For this review, take the finished solid that the model builds, in its own axes (mm). Face numbers are marked on the shaded views. A direction names the side the tool comes from. Coordinates: 2 decimals unless noted, no trailing zeros. Loops run counter-clockwise (first coordinate to the right, second up) from the corner with the lowest first, then second, coordinate; pieces in that order, holes last.
1. To check wall thickness, follow probe 1 along Y at (x, z) = (11, 56) (3 decimals); probe 2 along Y at (x, z) = (35, 37); probe 3 along X at (y, z) = (-11, -2) (3 decimals). State the ranges of each line that lie inside material, in increasing order.
2. Clearance check with flat-ended pins moving along their axes: P1, Ø20.5, axis at y = -5, z = 16, coming from the +X side (3 decimals); P2, Ø24, axis at x = 2.5, y = -32, coming from the +Z side (3 decimals); P3, Ø4, axis at x = 65, y = 24, coming from the -Z side; P4, Ø1, axis at x = 42, y = 30, coming from the -Z side. State where each tip first meets the part, or that it passes through.
3. Take a section at A-A, the plane y = -28. State the section outline as (x, z) points (3 decimals), then the cut area to 3 significant figures.
4. Machinability: for the marked faces 1, 2, 3, 4 and 5, which of the approach directions +Z, -Z, +X, -X, +Y, -Y give a long, thin tool a straight path to every point of the face, cutting with its end or side? Answer none if there is none.
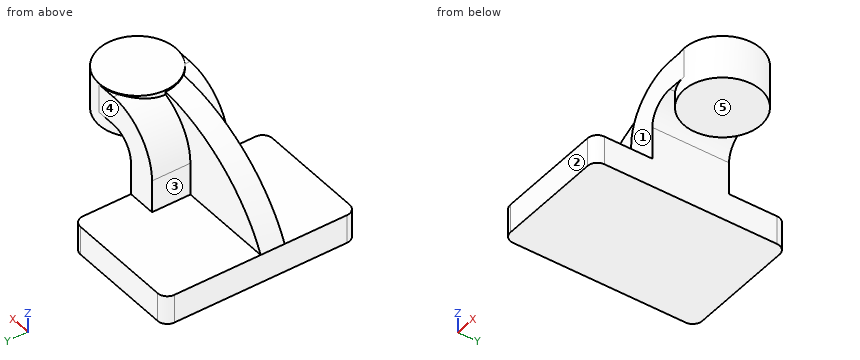
```python
from build123d import *

# Parameters (mm, degrees)
F1_DEPTH = 63.5
F2_DEPTH = 25.4
F3_DEPTH = 15.875
F5_R     = 6.35


with BuildPart() as f1:
    # F0 (on Front) → F1 (new body, symmetric)
    with BuildSketch(Plane.XZ):
        Polygon((-41.275, -9.525), (41.275, -9.525), (41.275, 9.525), (22.225, 9.525), (-41.275, 9.525), align=None)
    extrude(amount=F1_DEPTH, both=True)

    # F0 (on Front) → F2 (join, symmetric)
    with BuildSketch(Plane.XZ):
        with BuildLine():
            Line((22.225, 9.525), (41.275, 9.525))
            Line((41.275, 9.525), (41.275, 31.055324))
            ThreePointArc((41.275, 31.055324), (45.92468, 42.280644), (57.15, 46.930324))
            Line((57.15, 46.930324), (70.002963, 46.930324))
            Line((70.002963, 46.930324), (70.002963, 65.980324))
            Line((70.002963, 65.980324), (57.15, 65.980324))
            ThreePointArc((57.15, 65.980324), (32.454296, 55.751029), (22.225, 31.055324))
            Line((22.225, 31.055324), (22.225, 9.525))
        make_face()
    extrude(amount=F2_DEPTH, both=True)

    # F0 (on Front) → F3 (join)
    with BuildSketch(Plane.XZ):
        with BuildLine():
            add(Edge.make_bspline(
                [(-41.275, 9.525), (-26.659947, 40.76108), (10.355518, 66.98136), (57.15, 65.980324)],
                knots=[0, 0, 0, 0, 113.466666, 113.466666, 113.466666, 113.466666], degree=3))
            Line((-41.275, 9.525), (22.225, 9.525))
            Line((22.225, 9.525), (22.225, 31.055324))
            ThreePointArc((22.225, 31.055324), (32.454296, 55.751029), (57.15, 65.980324))
        make_face()
    extrude(amount=F3_DEPTH)

    # F0 (on Front) → F4 (revolve)
    with BuildSketch(Plane.XZ):
        Polygon((70.002963, 66.675), (70.002963, 65.980324), (70.002963, 46.930324), (70.002963, 38.1), (95.402963, 38.1), (95.402963, 66.675), align=None)
    revolve(axis=Axis((70.002963, 0, 52.3875), (0, 0, 1)))

    # F5
    f5_edges = [f1.edges().sort_by_distance(p)[0] for p in [
        (-41.275, -63.5, 0),
        (41.275, -63.5, 0),
        (-41.275, 63.5, 0),
        (41.275, 63.5, 0),
    ]]
    fillet(f5_edges, radius=F5_R)


solid = f1.part
```
Results list:
1. probe 1: y = -15.875 to 0
1. probe 2: y = -25.4 to 25.4
1. probe 3: x = -41.275 to 41.275
2. P1: stops at x = 41.275
2. P2: stops at z = 9.525
2. P3: stops at z = 38.1
2. P4: passes through
3. outline: (-41.275, -9.525) - (41.275, -9.525) - (41.275, 9.525) - (-41.275, 9.525) - close
3. area: 1,570 mm2
4. face 1: +Z, +X, -X, -Y
4. face 2: +Z, -Z, +X, -X, -Y
4. face 3: +Z, -X, +Y
4. face 4: +Z, +X, -X, +Y
4. face 5: -Z, +X, +Y, -Y
